```python
from build123d import *

# Parameters (mm, degrees)
SKETCH1_W           = 63.5
SKETCH1_H           = 28.575
BOSS_EXTRUDE1_DEPTH = 6.35
FILLET1_R           = 2.54
SKETCH2_W           = 33.02
SKETCH2_H           = 19.05
BOSS_EXTRUDE3_DEPTH = 33.02
SHELL1_START        = 6.35
SHELL1_OUTLINE_W    = 20.32
SHELL1_OUTLINE_H    = 6.35
SHELL1_DEPTH        = 26.67
SKETCH3_R           = 1.5875
CUT_EXTRUDE1_DEPTH  = 6.35
SKETCH4_W           = 3.175
SKETCH4_H           = 10.16
BOSS_EXTRUDE4_DEPTH = 19.05
FILLET4_R           = 1.27
FILLET6_R           = 3.175
SKETCH5_R           = 1.5875
CUT_EXTRUDE2_DEPTH  = 50.8
SKETCH8_W           = 3.175
SKETCH8_H           = 10.16
BOSS_EXTRUDE5_DEPTH = 19.05
SKETCH9_R           = 1.5875
CUT_EXTRUDE3_DEPTH  = 50.8
FILLET7_R           = 1.27
FILLET8_R           = 2.54
FILLET9_R           = 3.175


# Read off the part's stored shape, not the designer's step: Shell1
with BuildPart() as part:
    # Sketch1 → Boss-Extrude1 (new body)
    with BuildSketch(Plane(origin=(0, 0, 0), x_dir=(1, 0, 0), z_dir=(0, 1, 0))):
        Rectangle(SKETCH1_W, SKETCH1_H)
    extrude(amount=BOSS_EXTRUDE1_DEPTH)

    # Fillet1
    fillet1_edges = [part.edges().sort_by_distance(p)[0] for p in [
        (31.75, 3.175, 14.2875),
        (-31.75, 3.175, 14.2875),
        (-31.75, 3.175, -14.2875),
        (31.75, 3.175, -14.2875),
    ]]
    fillet(fillet1_edges, radius=FILLET1_R)

    # Sketch2 → Boss-Extrude3 (add)
    with BuildSketch(Plane(origin=(0, 6.35, 0), x_dir=(1, 0, 0), z_dir=(0, 1, 0))):
        Rectangle(SKETCH2_W, SKETCH2_H)
    extrude(amount=BOSS_EXTRUDE3_DEPTH)

    # Shell1 outline → Shell1 (cut)
    with BuildSketch(Plane(origin=(0, 0, 0), x_dir=(1, 0, 0), z_dir=(0, 1, 0)).offset(SHELL1_START)):
        Rectangle(SHELL1_OUTLINE_W, SHELL1_OUTLINE_H)
    extrude(amount=SHELL1_DEPTH, mode=Mode.SUBTRACT)

    # Sketch3 → Cut-Extrude1 (cut)
    with BuildSketch(Plane.XZ):
        with Locations(Location((-25.4, 0, 0), (0, 0, 270))):
            Circle(SKETCH3_R)
        with Locations(Location((25.4, 0, 0), (0, 0, 270))):
            Circle(SKETCH3_R)
    extrude(amount=-CUT_EXTRUDE1_DEPTH, mode=Mode.SUBTRACT)

    # Sketch4 → Boss-Extrude4 (add)
    with BuildSketch(Plane(origin=(0, 39.37, 0), x_dir=(1, 0, 0), z_dir=(0, 1, 0))):
        with Locations((-13.49375, 0)):
            Rectangle(SKETCH4_W, SKETCH4_H)
        with Locations((13.49375, 0)):
            Rectangle(SKETCH4_W, SKETCH4_H)
    extrude(amount=BOSS_EXTRUDE4_DEPTH)

    # Fillet4
    fillet4_edges = [part.edges().sort_by_distance(p)[0] for p in [
        (15.08125, 39.37, 0),
        (13.49375, 39.37, -5.08),
        (11.90625, 39.37, 0),
        (13.49375, 39.37, 5.08),
        (-15.08125, 39.37, 0),
        (-13.49375, 39.37, 5.08),
        (-11.90625, 39.37, 0),
        (-13.49375, 39.37, -5.08),
    ]]
    fillet(fillet4_edges, radius=FILLET4_R)

    # Fillet6
    fillet6_edges = [part.edges().sort_by_distance(p)[0] for p in [
        (13.49375, 58.42, -5.08),
        (13.49375, 58.42, 5.08),
        (-13.49375, 58.42, 5.08),
        (-13.49375, 58.42, -5.08),
    ]]
    fillet(fillet6_edges, radius=FILLET6_R)

    # Sketch5 → Cut-Extrude2 (cut)
    with BuildSketch(Plane(origin=(15.08125, 0, 0), x_dir=(0, 0, -1), z_dir=(1, 0, 0))):
        with Locations((0, 53.34)):
            Circle(SKETCH5_R)
    extrude(amount=-CUT_EXTRUDE2_DEPTH, mode=Mode.SUBTRACT)

    # Sketch8 → Boss-Extrude5 (add)
    with BuildSketch(Plane(origin=(0, 0, -9.525), x_dir=(-1, 0, 0), z_dir=(0, 0, -1))):
        with Locations((-13.49375, 22.86)):
            Rectangle(SKETCH8_W, SKETCH8_H)
        with Locations((13.49375, 22.86)):
            Rectangle(SKETCH8_W, SKETCH8_H)
    extrude(amount=BOSS_EXTRUDE5_DEPTH)

    # Sketch9 → Cut-Extrude3 (cut)
    with BuildSketch(Plane(origin=(15.08125, 0, 0), x_dir=(0, 0, -1), z_dir=(1, 0, 0))):
        with Locations(Location((23.495, 22.86, 0), (0, 0, 90))):
            Circle(SKETCH9_R)
    extrude(amount=-CUT_EXTRUDE3_DEPTH, mode=Mode.SUBTRACT)

    # Fillet7
    fillet7_edges = [part.edges().sort_by_distance(p)[0] for p in [
        (-15.08125, 22.86, -9.525),
        (-13.49375, 27.94, -9.525),
        (-11.90625, 22.86, -9.525),
        (-13.49375, 17.78, -9.525),
        (13.49375, 17.78, -9.525),
        (11.90625, 22.86, -9.525),
        (13.49375, 27.94, -9.525),
        (15.08125, 22.86, -9.525),
    ]]
    fillet(fillet7_edges, radius=FILLET7_R)

    # Fillet8
    fillet8_edges = [part.edges().sort_by_distance(p)[0] for p in [
        (16.51, 6.35, 0),
        (16.51, 22.86, 9.525),
        (0, 6.35, -9.525),
        (-16.51, 6.35, 0),
        (0, 6.35, 9.525),
        (-16.51, 22.86, 9.525),
        (0, 39.37, -9.525),
        (0, 39.37, 9.525),
    ]]
    fillet(fillet8_edges, radius=FILLET8_R)

    # Fillet9
    fillet9_edges = [part.edges().sort_by_distance(p)[0] for p in [
        (-13.49375, 27.94, -28.575),
        (-13.49375, 17.78, -28.575),
        (13.49375, 17.78, -28.575),
        (13.49375, 27.94, -28.575),
    ]]
    fillet(fillet9_edges, radius=FILLET9_R)


solid = part.part
```
Input: part model. Units: mm. Frame: model coordinates. A direction names the side the tool comes from. Give positions to 0.01 mm unless a question says otherwise; leave off trailing zeros. Order: outer loops, then holes, each group sorted by start corner. A loop starts at its lowest first (then second) coordinate and runs counter-clockwise, first axis right, second up. Notation, with made-up numbers: (31.25, 63) - (82.25, 63) arc R20 cw to (82.25, 94) - close; hole circle Ø4 at (21, 42). An arc over 180 degrees is marked (long way). Use a Markdown table: item, result.
(1) Section query B-B (y = 22.86). State how many separate pieces and enclosed holes the cut face has, then the cut area to 3 significant figures.
Computed values:
| item | result |
|---|---|
| separate pieces | 3 |
| enclosed holes | 1 |
| area | 599 mm2 |
(2) Pin query (flat end, axial travel): pin 1 (1 mm diameter, centred on x = 14.5, y = 46.5, fed in from -Z); pin 2 (2 mm diameter, centred on x = -12, y = 17.5, fed in from +Z) (3 decimals); pin 3 (5 mm diameter, centred on y = 10.5, z = 1.5, fed in from -X); pin 4 (4 mm diameter, centred on x = -25.4, z = 0, fed in from -Y). Return the tip coordinate at first contact, or that it passes through.
Computed values:
| item | result |
|---|---|
| pin 1 | stops at z = -5.08 |
| pin 2 | stops at z = 9.525 |
| pin 3 | stops at x = -16.67 |
| pin 4 | stops at y = 0 |
(3) Draft query along Z for faces 1 (the flat face through (-14, 48, -5.08)), 2 (the flat face through (-10.16, 19, 0)), 3 (the flat face through (-31.75, 3, 0)), 4 (the cylindrical face through (30.99, 3.22, 13.56)). Return one class per face: released by +Z, released by -Z, zero draft, split by the parting line, or undercut.
Computed values:
| item | result |
|---|---|
| face 1 | released by -Z |
| face 2 | undercut |
| face 3 | zero draft |
| face 4 | released by +Z |
(4) Section query D-D (y = 53.34). Output: boundary loops of the cut face in (x, z).
Computed values:
| item | result |
|---|---|
| outline | (-15.08, -5.08) - (-11.91, -5.08) - (-11.91, -1.59) - (-15.08, -1.59) - close; (-15.08, 1.59) - (-11.91, 1.59) - (-11.91, 5.08) - (-15.08, 5.08) - close; (11.91, -5.08) - (15.08, -5.08) - (15.08, -1.59) - (11.91, -1.59) - close; (11.91, 1.59) - (15.08, 1.59) - (15.08, 5.08) - (11.91, 5.08) - close |
(5) Section query C-C (z = -16.5). Output: boundary loops of the cut face in (x, y).
Computed values:
| item | result |
|---|---|
| outline | (-15.08, 17.78) - (-11.91, 17.78) - (-11.91, 27.94) - (-15.08, 27.94) - close; (11.91, 17.78) - (15.08, 17.78) - (15.08, 27.94) - (11.91, 27.94) - close |
(6) Section query A-A (x = -25.4). Output: boundary loops of the cut face in (y, z).
Computed values:
| item | result |
|---|---|
| outline | (0, -14.29) - (6.35, -14.29) - (6.35, -1.59) - (0, -1.59) - close; (0, 1.59) - (6.35, 1.59) - (6.35, 14.29) - (0, 14.29) - close |
(7) Line query: line 1 (Y direction, x = -12.9, z = 0); line 2 (Z direction, x = 13.25, y = 22.86) (1 decimal); line 3 (Z direction, x = -1, y = 25) (3 decimals). Output: solid intervals per line, ascending. Write a range as from..to.
Computed values:
| item | result |
|---|---|
| line 1 | y = 0..51.75, 54.93..58.42 |
| line 2 | z = -28.6..-25.1, -21.9..9.5 |
| line 3 | z = -9.525..-3.175, 3.175..9.525 |
(8) Access query for faces 5 (the flat face through (0, 3, -14.288)), 6 (the flat face through (11.906, 23, -20)), 7 (the flat face through (-11.906, 49, 0)), 8 (the flat face through (0, 19, -3.175)). Directions: +Z, -Z, +X, -X, +Y, -Y. A direction counts if a zero-diameter tool reaches every point of the face in a straight line with its end or side. Return the directions, or none.
Computed values:
| item | result |
|---|---|
| face 5 | -Z, +X, -X, -Y |
| face 6 | -Z, +Y |
| face 7 | +Z, -Z, +Y |
| face 8 | none |
